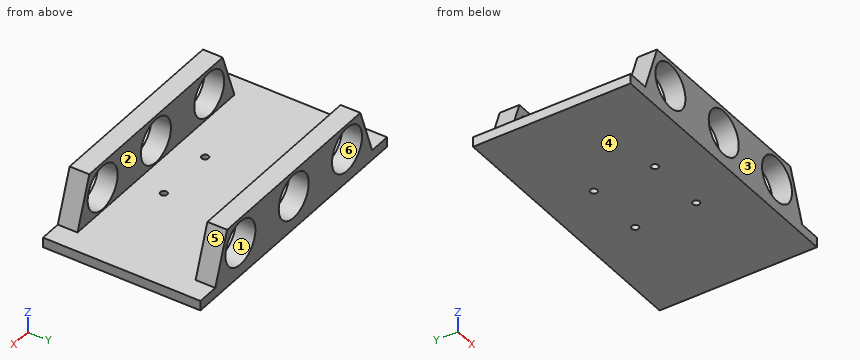
```python
from build123d import *

# Parameters (mm, degrees)
SKETCH_1_R          = 11.25
EXTRUDE_1_DEPTH     = 40
SKETCH_2_W          = 25
SKETCH_2_H          = 60
CUT_EXTRUDE1_DEPTH  = 149.176415127
SKETCH_3_R          = 1.75
CUT_EXTRUDE_1_DEPTH = 10


with BuildPart() as part:
    # Эскиз1 → Бобышка-Вытянуть1 (new, symmetric)
    with BuildSketch(Plane(origin=(0, 0, 0), x_dir=(1, 0, 0), z_dir=(0, 1, 0))):
        Polygon((-70, -2.5), (-58.870442851, -2.5), (-50, -27.5), (50, -27.5), (58.870442851, -2.5), (70, -2.5), (70, 2.5), (-70, 2.5), align=None)
        with Locations(Location((0, -14.5, 0), (0, 0, 270))):
            Circle(SKETCH_1_R, mode=Mode.SUBTRACT)
        with Locations(Location((40, -14.5, 0), (0, 0, 270))):
            Circle(SKETCH_1_R, mode=Mode.SUBTRACT)
        with Locations(Location((-40, -14.5, 0), (0, 0, 90))):
            Circle(SKETCH_1_R, mode=Mode.SUBTRACT)
    extrude(amount=EXTRUDE_1_DEPTH, both=True)

    # Эскиз2 → Cut-Extrude1 (cut, through all)
    with BuildSketch(Plane.ZY.offset(70)):
        with Locations((15, 0)):
            Rectangle(SKETCH_2_W, SKETCH_2_H)
    extrude(amount=-CUT_EXTRUDE1_DEPTH, mode=Mode.SUBTRACT)

    # Эскиз3 → Вырез-Вытянуть1 (cut)
    with BuildSketch(Plane(origin=(0, 0, -2.5), x_dir=(-1, 0, 0), z_dir=(0, 0, -1))):
        with Locations((-15.5, 15.5)):
            Circle(SKETCH_3_R)
        with Locations((15.5, 15.5)):
            Circle(SKETCH_3_R)
        with Locations((15.5, -15.5)):
            Circle(SKETCH_3_R)
        with Locations((-15.5, -15.5)):
            Circle(SKETCH_3_R)
    extrude(amount=-CUT_EXTRUDE_1_DEPTH, mode=Mode.SUBTRACT)


solid = part.part
```
Geometry check sheet. Reference: the model listing, model coordinates, mm. Face numbers are marked on the shaded views. A direction names the side the tool comes from. Coordinates: 2 decimals unless noted, no trailing zeros. Order: outer loops, then holes, each group sorted by start corner. A loop starts at its lowest first (then second) coordinate and runs counter-clockwise, first axis right, second up. Notation, with made-up numbers: M 78,4 L 100,4 A23 ccw 100,31 Z; hole C 85,19.5 d5. An arc over 180 degrees is marked long. Answer as a JSON object with one key per item and string values.
Q1. Cross-section at D-D on z = 16.5. Give the number of separate pieces and of enclosed holes in the cut face, and give its area (3 significant figures).
Results are:
{"separate pieces": "8", "enclosed holes": "0", "area": "828 mm²"}
Q2. Release check for a two-part mould opening along Z. For the marked faces 3, 4, 5 and 6 record: released by +Z, released by -Z, zero draft, split by the parting line, or undercut.
Results are:
{"face 3": "zero draft", "face 4": "released by -Z", "face 5": "released by +Z", "face 6": "undercut"}
Q3. Tool access check on the marked faces 1 and 2. Record the directions out of +Z, -Z, +X, -X, +Y, -Y that give a thin tool (end or side, any length) a straight path to the whole face; none if there is none.
Results are:
{"face 1": "+Y, -Y", "face 2": "+Z, +X, -X"}
Q4. Cross-section at B-B on y = -15.5. Record the cut outline in (x, z), and give its area (3 significant figures).
Results are:
{"outline": "M -70,-2.5 L -17.25,-2.5 L -17.25,2.5 L -70,2.5 Z; M -13.75,-2.5 L 13.75,-2.5 L 13.75,2.5 L -13.75,2.5 Z; M 17.25,-2.5 L 70,-2.5 L 70,2.5 L 17.25,2.5 Z", "area": "665 mm²"}
Q5. Depth check by flat-ended pin: pin 1 Ø5 at (x, y) = (-14.5, 15.5) entering from +Z; pin 2 Ø2 at (y, z) = (-30.5, 11) entering from +X. Enter the tip coordinate at first touch or a pass-through.
Results are:
{"pin 1": "stops at z = 2.5", "pin 2": "stops at x = 56.21"}
Q6. Scan lines: line 1 (Y direction, x = 15.5, z = -1.2); line 2 (X direction, y = 34, z = 14.5); line 3 (Y direction, x = -32.5, z = 4). Record each from-to range of solid material in increasing order.
Results are:
{"line 1": "y = -40 to -17.25, -13.75 to 13.75, 17.25 to 40", "line 2": "x = -54.61 to -51.25, -28.75 to -11.25, 11.25 to 28.75, 51.25 to 54.61", "line 3": "y = -40 to -30, 30 to 40"}
Q7. Cross-section at C-C on y = -31.5. Record the cut outline in (x, z), and give its area (3 significant figures).
Results are:
{"outline": "M -70,-2.5 L 70,-2.5 L 70,2.5 L 58.87,2.5 L 50,27.5 L -50,27.5 L -58.87,2.5 L -70,2.5 Z; hole C -40,14.5 d22.5; hole C 0,14.5 d22.5; hole C 40,14.5 d22.5", "area": "2,230 mm²"}
Q8. Cross-section at A-A on x = -15.5. Record the cut outline in (y, z).
Results are:
{"outline": "M -40,-2.5 L -17.25,-2.5 L -17.25,2.5 L -30,2.5 L -30,27.5 L -40,27.5 Z; M -13.75,-2.5 L 13.75,-2.5 L 13.75,2.5 L -13.75,2.5 Z; M 17.25,-2.5 L 40,-2.5 L 40,27.5 L 30,27.5 L 30,2.5 L 17.25,2.5 Z"}
